from build123d import *

# Parameters (mm, degrees)
EXTRUDE_START            = 9.5
SKETCH_1_R               = 35.986394748
EXTRUDE_1_DEPTH          = 19.1
SKETCH_1_3_R             = 19
CUT_EXTRUDE_1_DEPTH      = 52.789972136
EXTRUDE_START_2          = -12.6
SKETCH_1_4_R             = 37.5
EXTRUDE_2_DEPTH          = 3
CUT_EXTRUDE_2_DEPTH      = 55.509265267
CUT_EXTRUDE_2_DEPTH_BACK = 55.509265267
SKETCH_1_5_R             = 8.5
HOLE_WIZARD_M3_1_D       = 3.2


with BuildPart() as part:
    # ｽｹｯﾁ1 → ﾎﾞｽ - 押し出し1 (new body)
    with BuildSketch(Plane.XY.offset(EXTRUDE_START)):
        Circle(SKETCH_1_R)
    extrude(amount=-EXTRUDE_1_DEPTH)

    # ｽｹｯﾁ1<3> → ｶｯﾄ - 押し出し1 (cut, through all)
    with BuildSketch(Plane.XY):
        Circle(SKETCH_1_3_R)
    extrude(amount=CUT_EXTRUDE_1_DEPTH, mode=Mode.SUBTRACT)

    # ｽｹｯﾁ1<4> → ﾎﾞｽ - 押し出し2 (add)
    with BuildSketch(Plane.XY.offset(EXTRUDE_START_2)):
        Circle(SKETCH_1_4_R)
    extrude(amount=EXTRUDE_2_DEPTH)

    # ｽｹｯﾁ1<5> → ｶｯﾄ - 押し出し2 (cut, two sides: drawn at the far end of the back side and taken through both)
    with BuildSketch(Plane.XY.offset(-CUT_EXTRUDE_2_DEPTH_BACK)):
        Circle(SKETCH_1_5_R)
    extrude(amount=CUT_EXTRUDE_2_DEPTH + CUT_EXTRUDE_2_DEPTH_BACK, mode=Mode.SUBTRACT)

    # M3 すきま穴1 (through all)
    with Locations(Plane(origin=(0, 15, 0), x_dir=(1, 0, 0), z_dir=(0, 0, 1))):
        with Locations((0, 0), (-15, -15), (0, -30), (15, -15)):
            Hole(HOLE_WIZARD_M3_1_D / 2)


solid = part.part
CAD build for the part. Positions are in the model's coordinates, mm. A direction names the side the tool comes from. Coordinates: 2 decimals unless noted, no trailing zeros. Write each loop counter-clockwise with the first axis right and the second up, starting at its lowest first coordinate (ties: lowest second). Pieces come first, ordered by that corner, then holes. Notation, with made-up numbers: M 75.5,46 L 103.5,46 A26 ccw 103.5,63 Z; hole C 76,69.5 d8. An arc over 180 degrees is marked long. Answer as a JSON object with one key per item and string values. Group by question number.
1) Pin check, flat tips, straight feed: pin 1 Ø3 at (x, y) = (-15, 0) entering from -Z; pin 2 Ø2 at (y, z) = (-9.5, 0.5) entering from +X; pin 3 Ø4 at (x, y) = (15, 0) entering from -Z; pin 4 Ø11.5 at (x, y) = (-7.5, 4) entering from +Z. Stop position of each tip, or through.
2) Wall check: line 1 (Y direction, x = 0, z = -4.25); line 2 (Y direction, x = 0, z = 3); line 3 (X direction, y = -5.5, z = -1.25). Give the ranges that are in metal, low to high. Write a range as from..to.
3) Saw through at A-A (x = 0). Write the cut outline in (y, z), plus the area to 3 significant figures.
4) Mould opens along Y. For faces 1 (the face through (0.208, -13.414, -6.388)), 2 (the face through (-1, 9, -12.6)), 3 (the face through (16.606, -31.926, 0.084)) say: +Y half, -Y half, draft (parallel to the pull), parting line (faces both ways), or undercut.
5) Saw through at D-D (y = -15). Write the cut outline in (x, z), plus the area to 3 significant figures.
6) Tool access for faces 4 (the face through (8, -4, 0)), 5 (the face through (0.208, 16.586, -6.388)): list every direction of +Z, -Z, +X, -X, +Y, -Y with a clear straight run to the whole face (end or side of a thin tool).
7) Saw through at C-C (z = -5). Write the cut outline in (x, y), plus the area to 3 significant figures.
Values follow:
{
 "1": {"pin 1": "passes through", "pin 2": "stops at x = 34.97", "pin 3": "stops at z = -12.6", "pin 4": "stops at z = 0"},
 "2": {"line 1": "y = -35.99..-16.6, -13.4..-8.5, 8.5..13.4, 16.6..35.99", "line 2": "y = -35.99..-19, 19..35.99", "line 3": "x = -35.56..-6.48, 6.48..35.56"},
 "3": {"outline": "M -37.5,-12.6 L -16.6,-12.6 L -16.6,0 L -19,0 L -19,9.5 L -35.99,9.5 L -35.99,-9.6 L -37.5,-9.6 Z; M -13.4,-12.6 L -8.5,-12.6 L -8.5,0 L -13.4,0 Z; M 8.5,-12.6 L 13.4,-12.6 L 13.4,0 L 8.5,0 Z; M 16.6,-12.6 L 37.5,-12.6 L 37.5,-9.6 L 35.99,-9.6 L 35.99,9.5 L 19,9.5 L 19,0 L 16.6,0 Z", "area": "944 mm2"},
 "4": {"face 1": "undercut", "face 2": "draft", "face 3": "parting line"},
 "5": {"outline": "M -34.37,-12.6 L -1.6,-12.6 L -1.6,0 L -11.66,0 L -11.66,9.5 L -32.71,9.5 L -32.71,-9.6 L -34.37,-9.6 Z; M 1.6,-12.6 L 34.37,-12.6 L 34.37,-9.6 L 32.71,-9.6 L 32.71,9.5 L 11.66,9.5 L 11.66,0 L 1.6,0 Z", "area": "1,190 mm2"},
 "6": {"face 4": "+Z", "face 5": "+Z, -Z"},
 "7": {"outline": "C 0,0 d71.97; hole C -15,0 d3.2; hole C 0,0 d17; hole C 0,-15 d3.2; hole C 0,15 d3.2; hole C 15,0 d3.2", "area": "3,810 mm2"}
}
